Read the model definition and answer for the solid it produces. Units are mm, in the model's axes. A direction names the side the tool comes from. Coordinates: 2 decimals unless noted, no trailing zeros. Order: outer loops, then holes, each group sorted by start corner. A loop starts at its lowest first (then second) coordinate and runs counter-clockwise, first axis right, second up. Notation, with made-up numbers: (-8.75, -4) - (26.25, -4) arc R20 cw to (26.25, 18) - close; hole circle Ø1 at (30, 89). An arc over 180 degrees is marked (long way). Use one line per item in the form item = value. Start each with the question number.
from build123d import *

# Parameters (mm, degrees)
SKETCH1_W           = 30
SKETCH1_H           = 30
BOSS_EXTRUDE1_DEPTH = 1
SKETCH2_R           = 1
CUT_EXTRUDE1_DEPTH  = 2
SKETCH3_R           = 1
BOSS_EXTRUDE2_DEPTH = 2


with BuildPart() as part:
    # Sketch1 → Boss-Extrude1 (new body)
    with BuildSketch(Plane.XY):
        Rectangle(SKETCH1_W, SKETCH1_H)
    extrude(amount=BOSS_EXTRUDE1_DEPTH)

    # Sketch2 → Cut-Extrude1 (cut, through all)
    with BuildSketch(Plane.XY.offset(1)):
        with Locations((-13.14, 13.14)):
            Circle(SKETCH2_R)
        with Locations((13.14, 13.14)):
            Circle(SKETCH2_R)
        with Locations((13.14, -13.14)):
            Circle(SKETCH2_R)
        with Locations((-13.14, -13.14)):
            Circle(SKETCH2_R)
    extrude(amount=-CUT_EXTRUDE1_DEPTH, mode=Mode.SUBTRACT)

    # Sketch3 → Boss-Extrude2 (add)
    with BuildSketch(Plane.XY.offset(1)):
        Circle(SKETCH3_R)
    extrude(amount=BOSS_EXTRUDE2_DEPTH)


solid = part.part
Q1. Consider probe 1 along Y at (x, z) = (-13.14, 0.35); probe 2 along Z at (x, y) = (9.5, -10.25); probe 3 along X at (y, z) = (-0.25, 1.5). Determine where each line is inside the solid, lowest interval first.
Q2. Which of the six approach directions +Z, -Z, +X, -X, +Y, -Y give full straight-line access (tool end or side, diameter ignored) to faces 5 (the cylindrical face through (0, -1, 2)), 6 (the flat face through (15, -0.2, 0.5))?
Q3. A cutting plane is placed at A-A (x = 13.14). Give the vertices of the cut face in (y, z), then the cut area to 3 significant figures.
Q4. Given P1, Ø1.8, axis at x = 13.14, y = -13.14, coming from the +Z side; P2, Ø4, axis at x = 3, y = 6.5, coming from the +Z side, each flat-ended and moving along its own axis, determine where each tip first touches the part or whether it passes through.
Q5. A cutting plane is placed at D-D (x = 0). Give the vertices of the cut face in (y, z), then the cut area to 3 significant figures.
Q6. A cutting plane is placed at C-C (z = 2.35). Give the vertices of the cut face in (x, y).
Q7. For a pull along Y with two mould halves and no side action, classify faces 1 (the cylindrical face through (-12.68, -14.03, 0.51)), 2 (the flat face through (-0.2, 15, 0.5)), 3 (the flat face through (0, 0, 3)), 4 (the cylindrical face through (12.35, -13.75, 0.51)) as +Y half, -Y half, draft (parallel to the pull), parting line (faces both ways), or undercut.
Result sheet:
q1.probe_1 = -15 to -14.14, -12.14 to 12.14, 14.14 to 15
q1.probe_2 = 0 to 1
q1.probe_3 = -0.97 to 0.97
q2.face_5 = +Z
q2.face_6 = +Z, -Z, +X, +Y, -Y
q3.outline = (-15, 0) - (-14.14, 0) - (-14.14, 1) - (-15, 1) - close; (-12.14, 0) - (12.14, 0) - (12.14, 1) - (-12.14, 1) - close; (14.14, 0) - (15, 0) - (15, 1) - (14.14, 1) - close
q3.area = 26.0 mm^2
q4.P1 = through
q4.P2 = 1
q5.outline = (-15, 0) - (15, 0) - (15, 1) - (1, 1) - (1, 3) - (-1, 3) - (-1, 1) - (-15, 1) - close
q5.area = 34.0 mm^2
q6.outline = circle Ø2 at (0, 0)
q7.face_1 = undercut
q7.face_2 = +Y half
q7.face_3 = draft
q7.face_4 = undercut
